The model under review builds one solid part; all positions refer to its coordinate system, in mm. Give positions to 0.01 mm unless a question says otherwise; leave off trailing zeros. Loops run counter-clockwise (first coordinate to the right, second up) from the corner with the lowest first, then second, coordinate; pieces in that order, holes last. Notation, with made-up numbers: (86, 39.25) - (128, 39.25) arc R15 ccw to (128, 54.25) - close; hole circle Ø5 at (85, -11.75). An arc over 180 degrees is marked (long way). Answer as a JSON object with one key per item and string values.
from build123d import *

# Parameters (mm, degrees)
SKETCH1_W           = 112
SKETCH1_H           = 70
BOSS_EXTRUDE1_DEPTH = 2
FILLET1_R           = 3
SKETCH2_R           = 2.05
CUT_EXTRUDE1_DEPTH  = 3


with BuildPart() as part:
    # Sketch1 → Boss-Extrude1 (new body)
    with BuildSketch(Plane.XY):
        with Locations((-34.191460674, -27.067695099)):
            Rectangle(SKETCH1_W, SKETCH1_H)
    extrude(amount=BOSS_EXTRUDE1_DEPTH)

    # Fillet1
    fillet1_edges = [part.edges().sort_by_distance(p)[0] for p in [
        (-90.191460674, 7.932304901, 1),
        (21.808539326, 7.932304901, 1),
        (21.808539326, -62.067695099, 1),
        (-90.191460674, -62.067695099, 1),
    ]]
    fillet(fillet1_edges, radius=FILLET1_R)

    # Sketch2 → Cut-Extrude1 (cut)
    with BuildSketch(Plane.XY.offset(2)):
        with Locations((-84.272277823, -56.067695099)):
            Circle(SKETCH2_R)
        with Locations((-85.772277823, -39.067695099)):
            Circle(SKETCH2_R)
        with Locations((-85.772277823, -15.067695099)):
            Circle(SKETCH2_R)
        with Locations((-84.272277823, 1.932304901)):
            Circle(SKETCH2_R)
        with Locations((-60.272277823, 3.432304901)):
            Circle(SKETCH2_R)
        with Locations((-60.191460674, -57.567695099)):
            Circle(SKETCH2_R)
        with Locations((-34.231869249, -57.567695099)):
            Circle(SKETCH2_R)
        with Locations((-34.231869249, 3.432304901)):
            Circle(SKETCH2_R)
        with Locations((-8.191460674, 3.432304901)):
            Circle(SKETCH2_R)
        with Locations((-8.191460674, -57.567695099)):
            Circle(SKETCH2_R)
        with Locations((15.808539326, -56.067695099)):
            Circle(SKETCH2_R)
        with Locations((17.308539326, -39.067695099)):
            Circle(SKETCH2_R)
        with Locations((17.308539326, -15.067695099)):
            Circle(SKETCH2_R)
        with Locations((15.808539326, 1.932304901)):
            Circle(SKETCH2_R)
    extrude(amount=-CUT_EXTRUDE1_DEPTH, mode=Mode.SUBTRACT)


solid = part.part
Q1. Clearance check with a flat-ended pin moving along its axis: pin 1 Ø6.5 at (x, y) = (17.31, -39.07) entering from -Z. State where the tip first meets the part, or that it passes through.
Results:
{"pin 1": "stops at z = 0"}
Q2. Consider section A-A, the plane x = -8. State the section outline as (y, z) points.
Results:
{"outline": "(-62.07, 0) - (-59.61, 0) - (-59.61, 2) - (-62.07, 2) - close; (-55.53, 0) - (1.39, 0) - (1.39, 2) - (-55.53, 2) - close; (5.47, 0) - (7.93, 0) - (7.93, 2) - (5.47, 2) - close"}
Q3. To check wall thickness, follow probe 1 along Y at (x, z) = (-7, 0.85); probe 2 along X at (y, z) = (-56, 1.55); probe 3 along Y at (x, z) = (15, 1.55). State the ranges of each line that lie inside material, in increasing order. Write a range as [from, to].
Results:
{"probe 1": "y = [-62.07, -59.24], [-55.9, 1.76], [5.1, 7.93]", "probe 2": "x = [-90.19, -86.32], [-82.22, -61.51], [-58.87, -35.55], [-32.91, -9.51], [-6.87, 13.76], [17.86, 21.81]", "probe 3": "y = [-62.07, -57.95], [-54.18, 0.05], [3.82, 7.93]"}
Q4. The part is to be moulded in two halves that separate along Y. For faces 1 (the face through (20.953, 7.03, 1.014)), 2 (the face through (-89.3, -61.2, 1)), 3 (the face through (-86.32, 2.02, 1.01)), say which applies: +Y half, -Y half, draft (parallel to the pull), parting line (faces both ways), or undercut.
Results:
{"face 1": "+Y half", "face 2": "-Y half", "face 3": "undercut"}
Q5. Consider section B-B, the plane z = 0.95. State how many separate pieces and enclosed holes the cut face has, plus the area to 3 significant figures.
Results:
{"separate pieces": "1", "enclosed holes": "14", "area": "7,650 mm^2"}
